Geometry: final body of the model. Coordinates: model frame, mm. Face numbers are marked on the shaded views. A direction names the side the tool comes from. Coordinates: 2 decimals unless noted, no trailing zeros. Order: outer loops, then holes, each group sorted by start corner. A loop starts at its lowest first (then second) coordinate and runs counter-clockwise, first axis right, second up. Notation, with made-up numbers: (82, 70.5) - (131, 70.5) arc R18 cw to (131, 76.5) - close; hole circle Ø5 at (4.5, -18.5). An arc over 180 degrees is marked (long way). Use a Markdown table: item, result. Add a question column.
```python
from build123d import *

# Parameters (mm, degrees)
SKETCH2_W           = 101.6
SKETCH2_H           = 71.12
BOSS_EXTRUDE1_DEPTH = 76.2
SKETCH3_W           = 91.44
SKETCH3_H           = 60.96
CUT_EXTRUDE5_DEPTH  = 71.12
SKETCH5_R           = 3.302
CUT_EXTRUDE6_DEPTH  = 7.62
SKETCH7_R           = 5.08
CUT_EXTRUDE8_DEPTH  = 7.62
SKETCH8_W           = 20.32
SKETCH8_H           = 60.96
CUT_EXTRUDE9_DEPTH  = 7.62


with BuildPart() as part:
    # Sketch2 → Boss-Extrude1 (new body)
    with BuildSketch(Plane(origin=(0, 0, 0), x_dir=(1, 0, 0), z_dir=(0, 1, 0))):
        with Locations((6.092485814, -6.347086588)):
            Rectangle(SKETCH2_W, SKETCH2_H)
    extrude(amount=BOSS_EXTRUDE1_DEPTH)

    # Sketch3 → Cut-Extrude5 (cut)
    with BuildSketch(Plane(origin=(0, 76.2, 0), x_dir=(1, 0, 0), z_dir=(0, 1, 0))):
        with Locations((6.092485814, -6.347086588)):
            Rectangle(SKETCH3_W, SKETCH3_H)
    extrude(amount=-CUT_EXTRUDE5_DEPTH, mode=Mode.SUBTRACT)

    # Sketch5 → Cut-Extrude6 (cut)
    with BuildSketch(Plane.XY.offset(41.907086588)):
        with Locations((41.652485814, 15.24)):
            Circle(SKETCH5_R)
    extrude(amount=-CUT_EXTRUDE6_DEPTH, mode=Mode.SUBTRACT)

    # Sketch7 → Cut-Extrude8 (cut)
    with BuildSketch(Plane(origin=(0, 5.08, 0), x_dir=(1, 0, 0), z_dir=(0, 1, 0))):
        with Locations(Location((-12.957514186, -3.807086588, 0), (0, 0, 270))):
            Circle(SKETCH7_R)
        with Locations(Location((25.142485814, -6.347086588, 0), (0, 0, 270))):
            Circle(SKETCH7_R)
    extrude(amount=-CUT_EXTRUDE8_DEPTH, mode=Mode.SUBTRACT)

    # Sketch8 → Cut-Extrude9 (cut)
    with BuildSketch(Plane.ZY.offset(44.707514186)):
        with Locations((-11.432913412, 38.1)):
            Rectangle(SKETCH8_W, SKETCH8_H)
        with Locations((24.127086588, 38.1)):
            Rectangle(SKETCH8_W, SKETCH8_H)
    extrude(amount=-CUT_EXTRUDE9_DEPTH, mode=Mode.SUBTRACT)


solid = part.part
```
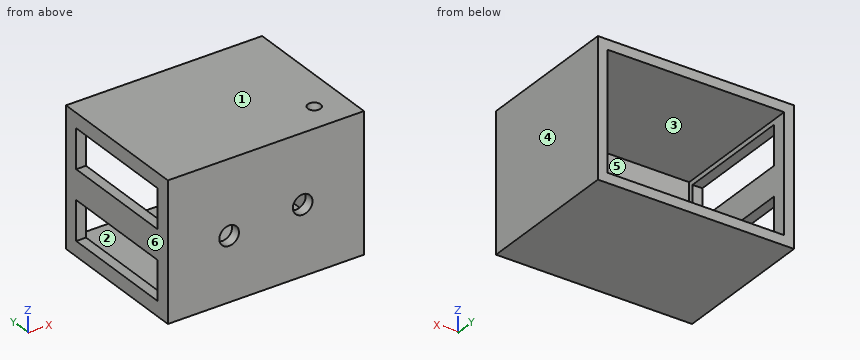
1) Line query: line 1 (X direction, y = 46.5, z = 0.5); line 2 (Z direction, x = -31.5, y = 61); line 3 (X direction, y = 15, z = 40). Output: solid intervals per line, ascending. Write a range as from..to.
2) Section query A-A (z = -8). Return the cut outline in (x, y), and give its area (3 significant figures).
3) First-contact query: pin 1 (4 mm diameter, centred on x = -42.5, z = 28.5, fed in from -Y); pin 2 (1.5 mm diameter, centred on y = 34, z = 15, fed in from -X); pin 3 (4 mm diameter, centred on x = 28, z = 24.5, fed in from +Y). Flat tips, straight axial feed; report the tip coordinate or a pass-through.
4) Section query B-B (y = 15.24). Return the cut outline in (x, z).
5) Draft query along X for the marked faces 1, 2, 3 and 4. Return one class per face: released by +X, released by -X, zero draft, split by the parting line, or undercut.
6) Section query C-C (x = 40.5). Return the cut outline in (y, z), and give its area (3 significant figures).
7) Access query for the marked faces 5 and 6. Directions: +Z, -Z, +X, -X, +Y, -Y. A direction counts if a zero-diameter tool reaches every point of the face in a straight line with its end or side. Return the directions, or none.
8) Section query D-D (y = 58.5). Return the cut outline in (x, z).
From the geometry:
| question | item | result |
|---|---|---|
| 1 | line 1 | x = -44.71..-39.63, 51.81..56.89 |
| 1 | line 2 | z = -29.21..-24.13, 36.83..41.91 |
| 1 | line 3 | x = -44.71..38.36, 44.95..56.89 |
| 2 | outline | (-44.71, 0) - (56.89, 0) - (56.89, 76.2) - (51.81, 76.2) - (51.81, 5.08) - (-39.63, 5.08) - (-39.63, 7.62) - (-44.71, 7.62) - close; (-44.71, 68.58) - (-39.63, 68.58) - (-39.63, 76.2) - (-44.71, 76.2) - close |
| 2 | area | 929 mm^2 |
| 3 | pin 1 | stops at y = 0 |
| 3 | pin 2 | stops at x = 51.81 |
| 3 | pin 3 | stops at y = 5.08 |
| 4 | outline | (-44.71, -29.21) - (56.89, -29.21) - (56.89, 41.91) - (44.95, 41.91) - (44.95, 36.83) - (51.81, 36.83) - (51.81, -24.13) - (-39.63, -24.13) - (-39.63, -21.59) - (-44.71, -21.59) - close; (-44.71, -1.27) - (-39.63, -1.27) - (-39.63, 13.97) - (-44.71, 13.97) - close; (-44.71, 34.29) - (-39.63, 34.29) - (-39.63, 36.83) - (38.35, 36.83) - (38.35, 41.91) - (-44.71, 41.91) - close |
| 5 | face 1 | zero draft |
| 5 | face 2 | undercut |
| 5 | face 3 | undercut |
| 5 | face 4 | released by +X |
| 6 | outline | (0, -29.21) - (76.2, -29.21) - (76.2, -24.13) - (5.08, -24.13) - (5.08, 36.83) - (12.15, 36.83) - (12.15, 41.91) - (0, 41.91) - close; (18.33, 36.83) - (76.2, 36.83) - (76.2, 41.91) - (18.33, 41.91) - close |
| 6 | area | 1,050 mm^2 |
| 7 | face 5 | +Y |
| 7 | face 6 | +Z, -Z, -X, +Y, -Y |
| 8 | outline | (-44.71, -29.21) - (56.89, -29.21) - (56.89, 41.91) - (-44.71, 41.91) - (-44.71, 34.29) - (-39.63, 34.29) - (-39.63, 36.83) - (51.81, 36.83) - (51.81, -24.13) - (-39.63, -24.13) - (-39.63, -21.59) - (-44.71, -21.59) - close; (-44.71, -1.27) - (-39.63, -1.27) - (-39.63, 13.97) - (-44.71, 13.97) - close |
